The listing builds one solid part. Answer for the finished solid, in the listing's coordinates (mm). A direction names the side the tool comes from. Coordinates: 2 decimals unless noted, no trailing zeros. Write each loop counter-clockwise with the first axis right and the second up, starting at its lowest first coordinate (ties: lowest second). Pieces come first, ordered by that corner, then holes. Notation, with made-up numbers: M 40.5,69.25 L 66.5,69.25 A25 cw 66.5,102.25 Z; hole C 19,27.25 d7. An arc over 180 degrees is marked long. Answer as a JSON object with one key per item and string values. Group by question number.
from build123d import *

# Parameters (mm, degrees)
ESQUISSE1_W             = 12.7
ESQUISSE1_H             = 25.4
BOSS_EXTRU_1_DEPTH      = 1.2
ESQUISSE2_R             = 1.0922
ESQUISSE2_R_2           = 0.6
ENL_V_MAT_EXTRU_1_DEPTH = 29.423405848
BOSS_EXTRU_2_START      = 0.02
ESQUISSE3_R             = 1
ESQUISSE3_R_2           = 0.6
ESQUISSE3_R_3           = 1.6922
ESQUISSE3_R_4           = 1.0922
ESQUISSE3_W             = 1.85
ESQUISSE3_H             = 1.85
BOSS_EXTRU_2_DEPTH      = 0.02
ESQUISSE4_R             = 1.6922
ESQUISSE4_R_2           = 1.0922
ESQUISSE4_R_3           = 1
ESQUISSE4_R_4           = 0.6
ESQUISSE4_W             = 1.8
ESQUISSE4_H             = 1.801050322
BOSS_EXTRU_3_DEPTH      = 0.02
ESQUISSE5_W             = 2.509277943
ESQUISSE5_H             = 2.515443245
ESQUISSE5_W_2           = 3.091420622
ESQUISSE5_H_2           = 3.048603163
ESQUISSE5_W_3           = 3.06104158
ESQUISSE5_H_3           = 3.068544132
ESQUISSE5_W_4           = 1.193610918
ESQUISSE5_H_4           = 2.854286977
ESQUISSE5_W_5           = 1.26351165
ESQUISSE5_H_5           = 2.853107199
ESQUISSE5_W_6           = 1.59060758
ESQUISSE5_H_6           = 2.920070631
BOSS_EXTRU_4_DEPTH      = 0.8
ESQUISSE6_W             = 1.618272423
ESQUISSE6_H             = 0.858257016
ESQUISSE6_W_2           = 1.550371274
ESQUISSE6_H_2           = 0.746748434
BOSS_EXTRU_5_DEPTH      = 0.6
BOSS_EXTRU_6_DEPTH      = 0.35


with BuildPart() as part:
    # Esquisse1 → Boss.-Extru.1 (new body)
    with BuildSketch(Plane(origin=(0, 0, 0), x_dir=(1, 0, 0), z_dir=(0, 1, 0))):
        with Locations((6.35, 12.7)):
            Rectangle(ESQUISSE1_W, ESQUISSE1_H)
    extrude(amount=BOSS_EXTRU_1_DEPTH)

    # Esquisse2 → Enlèv. mat.-Extru.1 (cut, through all)
    with BuildSketch(Plane(origin=(0, 1.2, 0), x_dir=(1, 0, 0), z_dir=(0, 1, 0))):
        with Locations(Location((2.54, 7.48, 0), (0, 0, 270))):
            Circle(ESQUISSE2_R)
        with Locations(Location((10.16, 2.4, 0), (0, 0, 270))):
            Circle(ESQUISSE2_R)
        with Locations(Location((6.35, 24.13, 0), (0, 0, 270))):
            Circle(ESQUISSE2_R_2)
        with Locations(Location((8.89, 24.13, 0), (0, 0, 270))):
            Circle(ESQUISSE2_R_2)
        with Locations(Location((11.43, 24.13, 0), (0, 0, 270))):
            Circle(ESQUISSE2_R_2)
        with Locations(Location((3.81, 24.13, 0), (0, 0, 270))):
            Circle(ESQUISSE2_R_2)
        with Locations(Location((1.27, 24.13, 0), (0, 0, 270))):
            Circle(ESQUISSE2_R_2)
        with Locations(Location((6.35, 21.59, 0), (0, 0, 270))):
            Circle(ESQUISSE2_R_2)
    extrude(amount=-ENL_V_MAT_EXTRU_1_DEPTH, mode=Mode.SUBTRACT)

    # Esquisse3 → Boss.-Extru.2 (add)
    # profile 1 of 8: a face of its own
    with BuildSketch(Plane(origin=(0, 1.2, 0), x_dir=(1, 0, 0), z_dir=(0, 1, 0)).offset(BOSS_EXTRU_2_START)):
        with Locations(Location((1.27, 24.13, 0), (0, 0, 90))):
            Circle(ESQUISSE3_R)
        with Locations(Location((1.27, 24.13, 0), (0, 0, 270))):
            Circle(ESQUISSE3_R_2, mode=Mode.SUBTRACT)
    # profile 2 of 8: a face of its own
    with BuildSketch(Plane(origin=(0, 1.2, 0), x_dir=(1, 0, 0), z_dir=(0, 1, 0)).offset(BOSS_EXTRU_2_START)):
        with Locations(Location((3.81, 24.13, 0), (0, 0, 90))):
            Circle(ESQUISSE3_R)
        with Locations(Location((3.81, 24.13, 0), (0, 0, 270))):
            Circle(ESQUISSE3_R_2, mode=Mode.SUBTRACT)
    # profile 3 of 8: a face of its own
    with BuildSketch(Plane(origin=(0, 1.2, 0), x_dir=(1, 0, 0), z_dir=(0, 1, 0)).offset(BOSS_EXTRU_2_START)):
        with Locations(Location((8.89, 24.13, 0), (0, 0, 90))):
            Circle(ESQUISSE3_R)
        with Locations(Location((8.89, 24.13, 0), (0, 0, 270))):
            Circle(ESQUISSE3_R_2, mode=Mode.SUBTRACT)
    # profile 4 of 8: a face of its own
    with BuildSketch(Plane(origin=(0, 1.2, 0), x_dir=(1, 0, 0), z_dir=(0, 1, 0)).offset(BOSS_EXTRU_2_START)):
        with Locations(Location((11.43, 24.13, 0), (0, 0, 90))):
            Circle(ESQUISSE3_R)
        with Locations(Location((11.43, 24.13, 0), (0, 0, 270))):
            Circle(ESQUISSE3_R_2, mode=Mode.SUBTRACT)
    # profile 5 of 8: a face of its own
    with BuildSketch(Plane(origin=(0, 1.2, 0), x_dir=(1, 0, 0), z_dir=(0, 1, 0)).offset(BOSS_EXTRU_2_START)):
        with Locations(Location((6.35, 21.59, 0), (0, 0, 90))):
            Circle(ESQUISSE3_R)
        with Locations(Location((6.35, 21.59, 0), (0, 0, 270))):
            Circle(ESQUISSE3_R_2, mode=Mode.SUBTRACT)
    # profile 6 of 8: a face of its own
    with BuildSketch(Plane(origin=(0, 1.2, 0), x_dir=(1, 0, 0), z_dir=(0, 1, 0)).offset(BOSS_EXTRU_2_START)):
        with Locations(Location((2.54, 7.48, 0), (0, 0, 90))):
            Circle(ESQUISSE3_R_3)
        with Locations(Location((2.54, 7.48, 0), (0, 0, 270))):
            Circle(ESQUISSE3_R_4, mode=Mode.SUBTRACT)
    # profile 7 of 8: a face of its own
    with BuildSketch(Plane(origin=(0, 1.2, 0), x_dir=(1, 0, 0), z_dir=(0, 1, 0)).offset(BOSS_EXTRU_2_START)):
        with Locations(Location((10.16, 2.4, 0), (0, 0, 90))):
            Circle(ESQUISSE3_R_3)
        with Locations(Location((10.16, 2.4, 0), (0, 0, 270))):
            Circle(ESQUISSE3_R_4, mode=Mode.SUBTRACT)
    # profile 8 of 8: a face of its own
    with BuildSketch(Plane(origin=(0, 1.2, 0), x_dir=(1, 0, 0), z_dir=(0, 1, 0)).offset(BOSS_EXTRU_2_START)):
        with Locations((6.35, 24.13)):
            Rectangle(ESQUISSE3_W, ESQUISSE3_H)
        with Locations(Location((6.35, 24.13, 0), (0, 0, 270))):
            Circle(ESQUISSE3_R_2, mode=Mode.SUBTRACT)
    extrude(amount=-BOSS_EXTRU_2_DEPTH)

    # Esquisse4 → Boss.-Extru.3 (add)
    # profile 1 of 8: a face of its own
    with BuildSketch(Plane(origin=(0, 0, 0), x_dir=(-1, 0, 0), z_dir=(0, -1, 0))):
        with Locations(Location((-2.54, 7.48, 0), (0, 0, 90))):
            Circle(ESQUISSE4_R)
        with Locations(Location((-2.54, 7.48, 0), (0, 0, 270))):
            Circle(ESQUISSE4_R_2, mode=Mode.SUBTRACT)
    # profile 2 of 8: a face of its own
    with BuildSketch(Plane(origin=(0, 0, 0), x_dir=(-1, 0, 0), z_dir=(0, -1, 0))):
        with Locations(Location((-10.16, 2.4, 0), (0, 0, 90))):
            Circle(ESQUISSE4_R)
        with Locations(Location((-10.16, 2.4, 0), (0, 0, 270))):
            Circle(ESQUISSE4_R_2, mode=Mode.SUBTRACT)
    # profile 3 of 8: a face of its own
    with BuildSketch(Plane(origin=(0, 0, 0), x_dir=(-1, 0, 0), z_dir=(0, -1, 0))):
        with Locations(Location((-6.35, 21.59, 0), (0, 0, 90))):
            Circle(ESQUISSE4_R_3)
        with Locations(Location((-6.35, 21.59, 0), (0, 0, 270))):
            Circle(ESQUISSE4_R_4, mode=Mode.SUBTRACT)
    # profile 4 of 8: a face of its own
    with BuildSketch(Plane(origin=(0, 0, 0), x_dir=(-1, 0, 0), z_dir=(0, -1, 0))):
        with Locations(Location((-8.89, 24.13, 0), (0, 0, 90))):
            Circle(ESQUISSE4_R_3)
        with Locations(Location((-8.89, 24.13, 0), (0, 0, 270))):
            Circle(ESQUISSE4_R_4, mode=Mode.SUBTRACT)
    # profile 5 of 8: a face of its own
    with BuildSketch(Plane(origin=(0, 0, 0), x_dir=(-1, 0, 0), z_dir=(0, -1, 0))):
        with Locations(Location((-11.43, 24.13, 0), (0, 0, 90))):
            Circle(ESQUISSE4_R_3)
        with Locations(Location((-11.43, 24.13, 0), (0, 0, 270))):
            Circle(ESQUISSE4_R_4, mode=Mode.SUBTRACT)
    # profile 6 of 8: a face of its own
    with BuildSketch(Plane(origin=(0, 0, 0), x_dir=(-1, 0, 0), z_dir=(0, -1, 0))):
        with Locations(Location((-3.81, 24.13, 0), (0, 0, 90))):
            Circle(ESQUISSE4_R_3)
        with Locations(Location((-3.81, 24.13, 0), (0, 0, 270))):
            Circle(ESQUISSE4_R_4, mode=Mode.SUBTRACT)
    # profile 7 of 8: a face of its own
    with BuildSketch(Plane(origin=(0, 0, 0), x_dir=(-1, 0, 0), z_dir=(0, -1, 0))):
        with Locations(Location((-1.27, 24.13, 0), (0, 0, 90))):
            Circle(ESQUISSE4_R_3)
        with Locations(Location((-1.27, 24.13, 0), (0, 0, 270))):
            Circle(ESQUISSE4_R_4, mode=Mode.SUBTRACT)
    # profile 8 of 8: a face of its own
    with BuildSketch(Plane(origin=(0, 0, 0), x_dir=(-1, 0, 0), z_dir=(0, -1, 0))):
        with Locations((-6.35, 24.13)):
            Rectangle(ESQUISSE4_W, ESQUISSE4_H)
        with Locations(Location((-6.35, 24.13, 0), (0, 0, 270))):
            Circle(ESQUISSE4_R_4, mode=Mode.SUBTRACT)
    extrude(amount=BOSS_EXTRU_3_DEPTH)

    # Esquisse5 → Boss.-Extru.4 (add)
    with BuildSketch(Plane.XZ):
        with Locations((4.605899052, -2.623946332)):
            Rectangle(ESQUISSE5_W, ESQUISSE5_H)
        with Locations((7.141800063, -7.814451049)):
            Rectangle(ESQUISSE5_W_2, ESQUISSE5_H_2)
        with Locations((9.635983842, -15.671495352)):
            Rectangle(ESQUISSE5_W_3, ESQUISSE5_H_3)
        with Locations((2.186822026, -14.841307754)):
            Rectangle(ESQUISSE5_W_4, ESQUISSE5_H_4)
        with Locations((2.491632252, -18.172449209)):
            Rectangle(ESQUISSE5_W_5, ESQUISSE5_H_5)
        with Locations((10.037187645, -21.174630377)):
            Rectangle(ESQUISSE5_W_6, ESQUISSE5_H_6)
    extrude(amount=BOSS_EXTRU_4_DEPTH)

    # Esquisse6 → Boss.-Extru.5 (add)
    with BuildSketch(Plane.XZ):
        Polygon((0.726627768, -2.066459052), (1.460485759, -2.066459052), (1.487334222, -3.552074009), (0.753476231, -3.552074009), align=None)
        Polygon((11.086694799, -7.026420932), (11.800319135, -7.026420932), (11.877628438, -8.554766384), (11.164004102, -8.554766384), align=None)
        Polygon((11.125349451, -10.627256859), (11.883196388, -10.627256859), (11.877628438, -12.112618353), (11.119781502, -12.112618353), align=None)
        Polygon((8.272243219, -10.085536784), (8.272243219, -10.819480111), (9.775079555, -10.871904634), (9.775079555, -10.137961308), align=None)
        Polygon((8.215171902, -11.68219873), (8.215171902, -12.455524532), (9.775079555, -12.461131564), (9.775079555, -11.687805762), align=None)
        Polygon((0.753476231, -12.068861631), (1.487334222, -12.068861631), (1.486411635, -10.570920499), (0.752553644, -10.570920499), align=None)
        Polygon((2.936295169, -12.12556249), (2.044305287, -12.12556249), (2.06534031, -10.526061527), (2.957330192, -10.526061527), align=None)
        Polygon((3.504383436, -12.12556249), (4.275795617, -12.12556249), (4.244730134, -10.579949827), (3.473317953, -10.579949827), align=None)
        Polygon((4.992958725, -12.174767916), (5.764370906, -12.174767916), (5.733305423, -10.629155253), (4.961893242, -10.629155253), align=None)
        Polygon((3.72603955, -22.142648569), (4.497451731, -22.142648569), (4.466386248, -20.597035906), (3.694974067, -20.597035906), align=None)
        with Locations((5.743109512, -19.098625419)):
            Rectangle(ESQUISSE6_W, ESQUISSE6_H)
        with Locations((10.517946357, -18.5651166)):
            Rectangle(ESQUISSE6_W_2, ESQUISSE6_H_2)
    extrude(amount=BOSS_EXTRU_5_DEPTH)

    # Esquisse7 → Boss.-Extru.6 (add)
    with BuildSketch(Plane.XZ):
        Polygon((4.982382693, -13.271878721), (4.982382693, -14.057624892), (6.524144098, -14.040635785), (6.524144098, -13.254889615), align=None)
        Polygon((5.057452454, -15.733592818), (6.59826695, -15.733592818), (6.58021053, -14.975223183), (5.039396034, -14.975223183), align=None)
        Polygon((5.048424244, -17.026123559), (5.048424244, -17.803582581), (6.581851825, -17.778567896), (6.581851825, -17.001108874), align=None)
        Polygon((1.179677832, -20.142278538), (1.179677832, -20.920603911), (2.727025883, -20.923704809), (2.727025883, -20.145379436), align=None)
        Polygon((1.134741003, -22.506266059), (1.122293095, -21.74319572), (2.689519452, -21.721611514), (2.701967359, -22.484681852), align=None)
    extrude(amount=BOSS_EXTRU_6_DEPTH)


solid = part.part
Item 1: A cutting plane is placed at D-D, the plane z = -12.75. Write down the section's boundary in (x, y), and give its area (3 significant figures).
Item 2: For a pull along Z with two mould halves and no side action, classify faces 1 (the face through (2.5, -0.8, -18.2)), 2 (the face through (6, 1, -25.4)), 3 (the face through (6, 1.2, -13)) as +Z half, -Z half, draft (parallel to the pull), parting line (faces both ways), or undercut.
Item 3: Flat-ended cylindrical pins translate along their axes: pin 1 Ø0.9 at (x, z) = (5.5, -13.5) entering from -Y; pin 2 Ø0.9 at (x, z) = (6, -19) entering from -Y; pin 3 Ø0.7 at (x, y) = (2.5, -0.5) entering from +Z. Find the tip coordinate at first contact, or state that the pin passes through.
Item 4: A cutting plane is placed at C-C, the plane z = -24.13. State how many separate pieces and enclosed holes the cut face has, and give its area (3 significant figures).
Item 5: A tool of negligible diameter and unlimited length cuts with its end or side. For faces 4 (the face through (9, -0.02, -3)), 5 (the face through (2, -0.8, -15)), from which of +Z, -Z, +X, -X, +Y, -Y can it reach the whole face along a straight path? Write none if from no direction.
Item 6: Consider L1, parallel to X at y = 0.75, z = -24.13; L2, parallel to Z at x = 4, y = -0.5; L3, parallel to Z at x = 8.75, y = -0.5. Determine where each line is inside the solid, lowest interval first. Write a range as from..to.
Answer:
{
 "1": {"outline": "M 0,0 L 12.7,0 L 12.7,1.2 L 0,1.2 Z", "area": "15.2 mm2"},
 "2": {"face 1": "draft", "face 2": "-Z half", "face 3": "undercut"},
 "3": {"pin 1": "y = -0.35", "pin 2": "y = -0.6", "pin 3": "z = -10.53"},
 "4": {"separate pieces": "6", "enclosed holes": "0", "area": "8.19 mm2"},
 "5": {"face 4": "+Z, +X, -Y", "face 5": "+Z, -Z, +X, -X, -Y"},
 "6": {"L1": "0..0.67, 1.87..3.21, 4.41..5.75, 6.95..8.29, 9.49..10.83, 12.03..12.7", "L2": "-22.14..-20.6, -12.13..-10.58, -3.88..-1.37", "L3": "-17.21..-14.14, -12.46..-11.68, -10.84..-10.1"}
}
